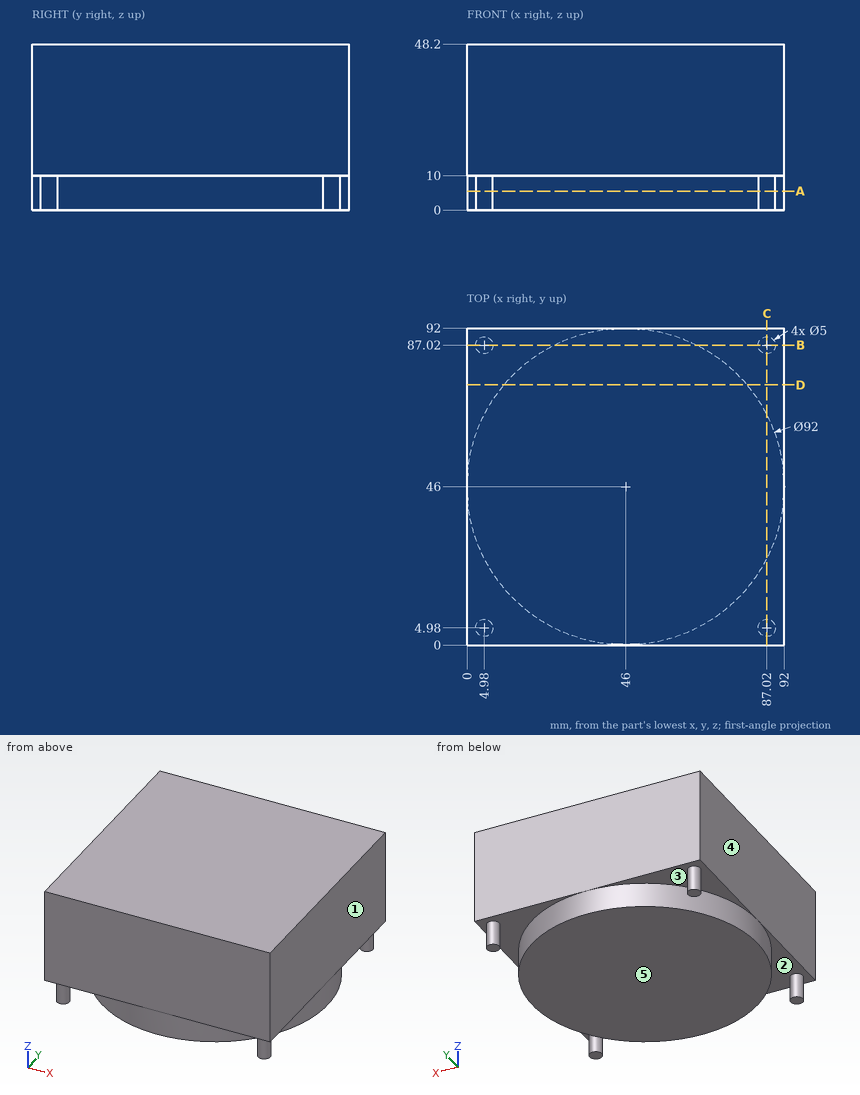
Verification items for this drawing (mm, ordinates from the low corner). A direction names the side the tool comes from. Give positions to 0.01 mm unless a question says otherwise; leave off trailing zeros. Loops run counter-clockwise (first coordinate to the right, second up) from the corner with the lowest first, then second, coordinate; pieces in that order, holes last. Notation, with made-up numbers: M 36.5,3.25 L 43.5,3.25 A17 cw 43.5,30.25 Z; hole C -7,-13 d11. An arc over 180 degrees is marked long. Answer as CSV lines item,"result".
Item 1: Release check for a two-part mould opening along X. For the marked faces 3, 4 and 5 record: pulls with the +X half, pulls with the -X half, needs draft (parallel to the pull), parting line crosses it, or undercut.
Values:
face 3,"undercut"
face 4,"pulls with the -X half"
face 5,"needs draft"
Item 2: Cross-section at B-B on y = 87.02. Record the cut outline in (x, z).
Values:
outline,"M 0,10 L 2.48,10 L 2.48,0 L 7.48,0 L 7.48,10 L 25.18,10 L 25.18,0 L 66.82,0 L 66.82,10 L 84.52,10 L 84.52,0 L 89.52,0 L 89.52,10 L 92,10 L 92,48.2 L 0,48.2 Z"
Item 3: Material ranges on line 1 (Z direction, x = 5, y = 70); line 2 (X direction, y = 73.5, z = 6); line 3 (X direction, y = 55.5, z = 7), recorded low to high.
Values:
line 1,"z = 10 to 48.2"
line 2,"x = 9.13 to 82.87"
line 3,"x = 0.99 to 91.01"
Item 4: Access from +Z, -Z, +X, -X, +Y, -Y to the whole of each face (thin tool, end or side, straight path). Record for the marked faces 1 and 2.
Values:
face 1,"+Z, -Z, +X, +Y, -Y"
face 2,"-Z"
Item 5: Cross-section at D-D on y = 75.5. Record the cut outline in (x, z).
Values:
outline,"M 0,10 L 10.7,10 L 10.7,0 L 81.3,0 L 81.3,10 L 92,10 L 92,48.2 L 0,48.2 Z"
Item 6: Cross-section at A-A on z = 5.5. Record the cut outline in (x, y).
Values:
outline,"C 46,46 d92; C 4.98,4.98 d5; C 4.98,87.02 d5; C 87.02,4.98 d5; C 87.02,87.02 d5"
